Part model, mm, in its own coordinate system. Give positions to 0.01 mm unless a question says otherwise; leave off trailing zeros. Write each loop counter-clockwise with the first axis right and the second up, starting at its lowest first coordinate (ties: lowest second). Pieces come first, ordered by that corner, then holes. Notation, with made-up numbers: (70.5, 8.25) - (85.5, 8.25) arc R28 cw to (85.5, 39.25) - close; hole circle Ø9 at (-9, 62.5). An arc over 180 degrees is marked (long way). Answer as a JSON object with one key per item and string values. Group by question number.
```python
from build123d import *

# Parameters (mm, degrees)
F1_DEPTH = 55.372


with BuildPart() as f1:
    # F0 (on Top) → F1 (new body)
    with BuildSketch(Plane.XY):
        Polygon((39.90279, -19.511992), (42.626367, -12.487726), (44.123662, -5.10421), (44.351599, 2.426144), (43.303621, 9.886703), (41.009877, 17.062839), (37.536354, 23.748109), (32.982977, 29.750188), (27.480741, 34.896409), (21.187934, 39.038724), (14.285588, 42.057965), (6.972273, 43.867276), (-0.541623, 44.414605), (-8.039937, 43.684207), (-15.306956, 41.697093), (-22.133623, 38.51043), (-28.323545, 34.215892), (-33.698651, 28.937026), (-38.104307, 22.825693), (-41.413772, 16.057707), (-43.531839, 8.82777), (-44.397573, 1.343874), (-43.98607, -6.178682), (-42.309168, -13.52349), (-39.415109, -20.479251), (-35.387148, -26.845861), (-30.341164, -32.440165), (-24.422319, -37.101224), (-17.800889, -40.694949), (-10.66736, -43.117954), (-3.22695, -44.300534), (4.306293, -44.208668), (11.715652, -42.845), (18.787973, -40.248758), (25.319799, -36.494634), (31.12322, -31.690625), (36.031282, -25.974934), align=None)
    extrude(amount=F1_DEPTH)


solid = f1.part
```
1) Band-saw the part on B-B (y = -8.5). List the corners of the cut face in (x, z), plus the area to 3 significant figures.
2) Drop flat-ended pins along their axis: P1, Ø2, axis at x = 9.5, z = 16.5, coming from the +Y side; P2, Ø5, axis at x = 3.5, y = -26.5, coming from the -Z side; P3, Ø10, axis at x = 26.5, z = 11.5, coming from the +Y side; P4, Ø12, axis at x = -8, z = 23.5, coming from the +Y side. Give the stop position or say it passes through.
3) Probe line 1 (Y direction, x = 23.5, z = 49.5); line 2 (Y direction, x = 37, z = 49); line 3 (X direction, y = 30.5, z = 11). List the from-to ranges inside material, lowest first.
4) Band-saw the part on A-A (x = 13). List the corners of the cut face in (y, z), plus the area to 3 significant figures.
Verdict:
{
 "1": {"outline": "(-43.46, 0) - (43.44, 0) - (43.44, 55.37) - (-43.46, 55.37) - close", "area": "4,810 mm2"},
 "2": {"P1": "y = 43.49", "P2": "z = 0", "P3": "y = 38.83", "P4": "y = 44.27"},
 "3": {"line 1": "-37.54 to 37.52", "line 2": "-24.36 to 24.46", "line 3": "-32.11 to 32.18"},
 "4": {"outline": "(-42.37, 0) - (42.38, 0) - (42.38, 55.37) - (-42.37, 55.37) - close", "area": "4,690 mm2"}
}
